Part model, mm, in its own coordinate system. A direction names the side the tool comes from. Round coordinates to 2 decimals unless told otherwise and drop trailing zeros. Loops run counter-clockwise (first coordinate to the right, second up) from the corner with the lowest first, then second, coordinate; pieces in that order, holes last. Notation, with made-up numbers: M 44.25,23.25 L 94.25,23.25 A19 cw 94.25,47.25 Z; hole C 51,19 d6. An arc over 180 degrees is marked long. Write each question's results on one line, items separated by ' | '.
from build123d import *

# Parameters (mm, degrees)
BOSS_EXTRUDE1_DEPTH = 13
SKETCH2_R           = 2.25
CUT_EXTRUDE1_DEPTH  = 3
SKETCH3_R           = 2
BOSS_EXTRUDE3_DEPTH = 3
BOSS_EXTRUDE4_START = 3
SKETCH4_R           = 2
BOSS_EXTRUDE4_DEPTH = 3
CUT_EXTRUDE2_DEPTH  = 3.5
CUT_EXTRUDE3_START  = -3.5
CUT_EXTRUDE3_DEPTH  = 3.5
FILLET1_R           = 6.5
SKETCH7_R           = 3.9
CUT_EXTRUDE4_DEPTH  = 60.076221951
CUT_EXTRUDE5_START  = -2
CUT_EXTRUDE5_DEPTH  = 2


with BuildPart() as part:
    # Sketch1 → Boss-Extrude1 (new body)
    with BuildSketch(Plane.XY):
        Polygon((3, 0), (3, 25), (36, 25), (36, 0), (39, 0), (39, 31), (35.5, 31), (35.5, 45), (3.5, 45), (3.5, 31), (0, 31), (0, 0), align=None)
    extrude(amount=BOSS_EXTRUDE1_DEPTH)

    # Sketch2 → Cut-Extrude1 (cut)
    with BuildSketch(Plane.ZY):
        with Locations((6.5, 5.293988539)):
            Circle(SKETCH2_R)
    extrude(amount=-CUT_EXTRUDE1_DEPTH, mode=Mode.SUBTRACT)

    # Sketch3 → Boss-Extrude3 (add)
    with BuildSketch(Plane.ZY.offset(-3.5)):
        with Locations(Location((6.5, 38.5, 0), (0, 0, 180))):
            Circle(SKETCH3_R)
    extrude(amount=BOSS_EXTRUDE3_DEPTH)

    # Sketch4 → Boss-Extrude4 (add)
    with BuildSketch(Plane(origin=(35.5, 0, 0), x_dir=(0, 0, -1), z_dir=(1, 0, 0)).offset(BOSS_EXTRUDE4_START)):
        with Locations((-6.5, 38.5)):
            Circle(SKETCH4_R)
    extrude(amount=-BOSS_EXTRUDE4_DEPTH)

    # Sketch5 → Cut-Extrude2 (cut)
    with BuildSketch(Plane.ZY):
        with BuildLine():
            Line((0, 24.5), (0, 34.231050233))
            Line((0, 34.231050233), (13, 34.231050233))
            Line((13, 34.231050233), (13, 24.5))
            ThreePointArc((13, 24.5), (6.5, 31), (0, 24.5))
        make_face()
    extrude(amount=-CUT_EXTRUDE2_DEPTH, mode=Mode.SUBTRACT)

    # Sketch6 → Cut-Extrude3 (cut)
    with BuildSketch(Plane(origin=(39, 0, 0), x_dir=(0, 0, -1), z_dir=(1, 0, 0)).offset(CUT_EXTRUDE3_START)):
        with BuildLine():
            Line((-13, 24.5), (-13, 34.712302794))
            Line((-13, 34.712302794), (0, 34.712302794))
            Line((0, 34.712302794), (0, 24.5))
            ThreePointArc((0, 24.5), (-6.5, 31), (-13, 24.5))
        make_face()
    extrude(amount=CUT_EXTRUDE3_DEPTH, mode=Mode.SUBTRACT)

    # Fillet1
    fillet1_edges = [part.edges().sort_by_distance(p)[0] for p in [
        (37.5, 0, 13),
        (37.5, 0, 0),
        (1.5, 0, 0),
        (1.5, 0, 13),
        (19.5, 45, 0),
        (19.5, 45, 13),
    ]]
    fillet(fillet1_edges, radius=FILLET1_R - 0.0001)  # a hair under: the kernel refuses the full size

    # Sketch7 → Cut-Extrude4 (cut, through all)
    with BuildSketch(Plane.ZY.offset(-36)):
        with Locations(Location((6.5, 5.293988539, 0), (0, 0, 270))):
            Circle(SKETCH7_R)
    extrude(amount=-CUT_EXTRUDE4_DEPTH, mode=Mode.SUBTRACT)

    # Sketch8 → Cut-Extrude5 (cut)
    with BuildSketch(Plane(origin=(39, 0, 0), x_dir=(0, 0, -1), z_dir=(1, 0, 0)).offset(CUT_EXTRUDE5_START)):
        with BuildLine():
            Line((-2.617023822, 5.657988539), (-4.010912706, 20.527321872))
            ThreePointArc((-4.010912706, 20.527321872), (-6.5, 22.793988539), (-8.989087294, 20.527321872))
            Line((-8.989087294, 20.527321872), (-10.382976178, 5.657988539))
            ThreePointArc((-10.382976178, 5.657988539), (-6.5, 1.393988539), (-2.617023822, 5.657988539))
        make_face()
    extrude(amount=CUT_EXTRUDE5_DEPTH, mode=Mode.SUBTRACT)


solid = part.part
Item 1: Band-saw the part on A-A on z = 9.75. Give the cut face in (x, y), and give its area (3 significant figures).
Filled sheet:
outline: M 0,0.87 L 3,0.87 L 3,25 L 36,25 L 36,7.45 L 37,7.45 L 37,12.41 L 39,12.41 L 39,30.13 L 35.5,30.13 L 35.5,44.13 L 3.5,44.13 L 3.5,30.13 L 0,30.13 Z; M 36,0.87 L 39,0.87 L 39,3.14 L 36,3.14 Z | area: 770 mm^2
Item 2: Wall check: L1, parallel to Y at x = 37.7, z = 6.5; L2, parallel to Y at x = 2.15, z = 6.5; L3, parallel to X at y = 5, z = 1. Give the ranges that are in metal, low to high.
Filled sheet:
L1: 0 to 1.39, 22.79 to 31, 36.5 to 40.5 | L2: 0 to 3.04, 7.54 to 31, 36.5 to 40.5 | L3: 0 to 3, 36 to 39
Item 3: Band-saw the part on D-D on z = 1. Give the cut face in (x, y).
Filled sheet:
outline: M 0,3.04 L 3,3.04 L 3,25 L 36,25 L 36,3.04 L 39,3.04 L 39,27.96 L 35.5,27.96 L 35.5,41.96 L 3.5,41.96 L 3.5,27.96 L 0,27.96 Z
Item 4: Two-plate mould, pull along X, no slides. Class faces 1 (the flat face through (19, 25, 6)), 2 (the flat face through (35.5, 35, 6)), 3 (the flat face through (36, 15, 6)), 4 (the flat face through (37.986, 12.989, 3.304)): +X half, -X half, draft (parallel to the pull), parting line (faces both ways), or undercut.
Filled sheet:
face 1: undercut | face 2: +X half | face 3: undercut | face 4: draft
Item 5: Band-saw the part on C-C on y = 34. Give the cut face in (x, z), and give its area (3 significant figures).
Filled sheet:
outline: M 3.5,0 L 35.5,0 L 35.5,13 L 3.5,13 Z | area: 416 mm^2
Item 6: Which spindle directions (+Z, -Z, +X, -X, +Y, -Y) get a long thin tool onto all of the face, cutting with end or side? Do faces 5 (the flat face through (0.5, 38, 7)), 6 (the flat face through (37, 14, 7)), 7 (the cylindrical face through (2.021, 40.452, 6.934)). Say none if no direction does.
Filled sheet:
face 5: +Z, -Z, -X, +Y | face 6: +X | face 7: -X
Item 7: Drop flat-ended pins along their axis: P1, Ø4, axis at y = 36.5, z = 4.5, coming from the +X side; P2, Ø2, axis at y = 38, z = 5.5, coming from the -X side; P3, Ø4, axis at x = 25, z = 3.5, coming from the -Y side. Give the stop position or say it passes through.
Filled sheet:
P1: x = 38.5 | P2: x = 0.5 | P3: y = 25
